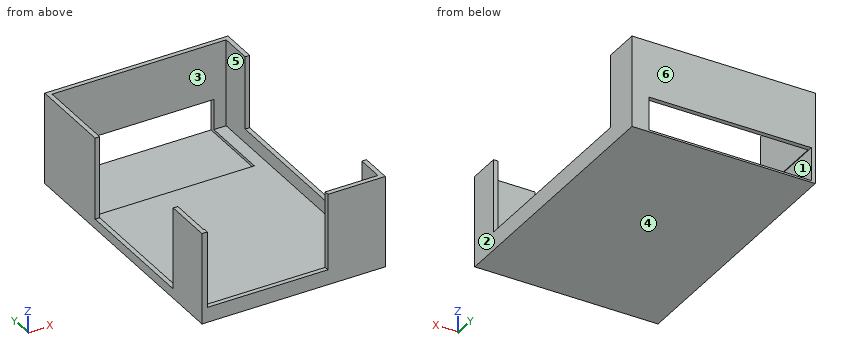
```python
from build123d import *

# Parameters (mm, degrees)
F0_W      = 63.5
F0_H      = 92.202
F1_DEPTH  = 31.75
F2_T      = -1.5875
F3_W      = 68.475886
F3_H      = 25.4
F4_DEPTH  = 25.4
F5_W      = 41.793442
F5_H      = 26.501633
F6_DEPTH  = 25.4
F7_W      = 45.800777
F7_H      = 28.45159
F8_DEPTH  = 25.4
F9_W      = 56.269303
F9_H      = 11.544435
F10_DEPTH = 25.4


with BuildPart() as f1:
    # F0 (on Top) → F1 (new body)
    with BuildSketch(Plane.XY):
        with Locations((2.364983, -4.317552)):
            Rectangle(F0_W, F0_H)
    extrude(amount=F1_DEPTH)

    # F2
    f2_openings = [f1.faces().sort_by_distance(p)[0] for p in [
        (2.364983, -4.317552, 31.75),
    ]]
    offset(amount=F2_T, openings=f2_openings)

    # F3 (on face) → F4 (cut)
    with BuildSketch(Plane.YZ.offset(34.114983)):
        with Locations((-5.154495, 19.05)):
            Rectangle(F3_W, F3_H)
    extrude(amount=-F4_DEPTH, mode=Mode.SUBTRACT)

    # F5 (on face) → F6 (cut)
    with BuildSketch(Plane.XZ.offset(50.418552)):
        with Locations((-6.639066, 18.499184)):
            Rectangle(F5_W, F5_H)
    extrude(amount=-F6_DEPTH, mode=Mode.SUBTRACT)

    # F7 (on face) → F8 (cut)
    with BuildSketch(Plane(origin=(-29.385017, 0, 0), x_dir=(0, -1, 0), z_dir=(-1, 0, 0))):
        with Locations((10.649152, 17.524205)):
            Rectangle(F7_W, F7_H)
    extrude(amount=-F8_DEPTH, mode=Mode.SUBTRACT)

    # F9 (on face) → F10 (cut)
    with BuildSketch(Plane(origin=(0, 41.783448, 0), x_dir=(-1, 0, 0), z_dir=(0, 1, 0))):
        with Locations((-0.107144, 6.392072)):
            Rectangle(F9_W, F9_H)
    extrude(amount=-F10_DEPTH, mode=Mode.SUBTRACT)


solid = f1.part
```
Geometry check sheet. Reference: the model listing, model coordinates, mm. Face numbers are marked on the shaded views. A direction names the side the tool comes from. Coordinates: 2 decimals unless noted, no trailing zeros. Write each loop counter-clockwise with the first axis right and the second up, starting at its lowest first coordinate (ties: lowest second). Pieces come first, ordered by that corner, then holes. Notation, with made-up numbers: M 50,58.25 L 61,58.25 A32 cw 61,93.25 Z; hole C 38,44.5 d6. An arc over 180 degrees is marked long. One line per item, written item: value. Start each with the question number.
(1) Sectioned sample at C-C, the plane y = -43.5. Enter the section's corners in (x, z), and give its area (3 significant figures).
(2) Sectioned sample at A-A, the plane z = 18.5. Enter the section's corners in (x, y), and give its area (3 significant figures).
(3) Release check for a two-part mould opening along Y. For the marked faces 4, 5 and 6 record: released by +Y, released by -Y, zero draft, split by the parting line, or undercut.
(4) Sectioned sample at D-D, the plane x = 6. Enter the section's corners in (y, z), and give its area (3 significant figures).
(5) Tool access check on the marked faces 1, 2 and 3. Record the directions out of +Z, -Z, +X, -X, +Y, -Y that give a thin tool (end or side, any length) a straight path to the whole face; none if there is none.
(6) Scan lines: line 1 along X through (y, z) = (-43, 18.5); line 2 along X through (y, z) = (28, 4); line 3 along Y through (x, z) = (19, 24). Record each from-to range of solid material in increasing order. Write a range as [from, to].
(7) Sectioned sample at B-B, the plane x = 22.5. Enter the section's corners in (y, z).
(8) Depth check by flat-ended pin: pin 1 (0.8 mm diameter, centred on x = -2, y = -50, fed in from +Z); pin 2 (2 mm diameter, centred on y = 15.5, z = 25.5, fed in from +X); pin 3 (0.5 mm diameter, centred on x = 33.5, y = -10, fed in from +Z). Enter the tip coordinate at first touch or a pass-through.
Filled sheet:
1. outline: M -29.39,0 L 34.11,0 L 34.11,31.75 L 32.53,31.75 L 32.53,1.59 L -27.8,1.59 L -27.8,31.75 L -29.39,31.75 Z
1. area: 197 mm²
2. outline: M -29.39,-50.42 L -27.54,-50.42 L -27.54,-48.83 L -27.8,-48.83 L -27.8,-33.55 L -29.39,-33.55 Z; M -29.39,12.25 L -27.8,12.25 L -27.8,40.2 L 32.53,40.2 L 32.53,29.08 L 34.11,29.08 L 34.11,41.78 L -29.39,41.78 Z; M 14.26,-50.42 L 34.11,-50.42 L 34.11,-39.39 L 32.53,-39.39 L 32.53,-48.83 L 14.26,-48.83 Z
2. area: 237 mm²
3. face 4: zero draft
3. face 5: undercut
3. face 6: released by +Y
4. outline: M -50.42,0 L 41.78,0 L 41.78,0.62 L 16.38,0.62 L 16.38,1.59 L -48.83,1.59 L -48.83,5.25 L -50.42,5.25 Z; M 40.2,12.16 L 41.78,12.16 L 41.78,31.75 L 40.2,31.75 Z
4. area: 159 mm²
5. face 1: +Y
5. face 2: +Z, -Z, +X, +Y, -Y
5. face 3: +Z
6. line 1: [-29.39, -27.8], [32.53, 34.11]
6. line 2: [-29.39, -28.03], [32.53, 34.11]
6. line 3: [-50.42, -48.83], [40.2, 41.78]
7. outline: M -50.42,0 L 41.78,0 L 41.78,0.62 L 16.38,0.62 L 16.38,1.59 L -48.83,1.59 L -48.83,31.75 L -50.42,31.75 Z; M 40.2,12.16 L 41.78,12.16 L 41.78,31.75 L 40.2,31.75 Z
8. pin 1: z = 5.25
8. pin 2: x = -27.8
8. pin 3: z = 6.35
